Check sheet for the modelled part. Datum: model origin and axes. Units: mm. A direction names the side the tool comes from. Coordinates: 2 decimals unless noted, no trailing zeros. Loops run counter-clockwise (first coordinate to the right, second up) from the corner with the lowest first, then second, coordinate; pieces in that order, holes last. Notation, with made-up numbers: M -25.5,77.25 L 22.5,77.25 A11 ccw 22.5,96.25 Z; hole C 8.25,3.5 d10. An arc over 180 degrees is marked long. Return JSON: item names as keys, results as strings.
from build123d import *

# Parameters (mm, degrees)
PAD003_DEPTH    = 30
SKETCH011_R     = 4.25
PAD004_DEPTH    = 2
SKETCH012_R     = 4.25
PAD005_DEPTH    = 2
SKETCH008_R     = 2.5
POCKET001_DEPTH = 28.501
SKETCH009_R     = 4.75
POCKET002_DEPTH = 28.501
SKETCH010_R     = 2.5
POCKET003_DEPTH = 48.111


with BuildPart() as part:
    # Sketch007 → Pad003 (new body, symmetric)
    with BuildSketch(Plane(origin=(0, 0, 10), x_dir=(0, 1, 0), z_dir=(1, 0, 0))):
        with BuildLine():
            Line((-12, 6.09), (-28.5, 6.09))
            Line((-28.5, 6.09), (-28.5, 14.09))
            Line((-28.5, 14.09), (-19.722169, 14.09))
            ThreePointArc((-14.09, 19.722169), (-17.656854, 17.656854), (-19.722169, 14.09))
            Line((-14.09, 19.722169), (-14.09, 34.02))
            ThreePointArc((0, 48.11), (-9.963135, 43.983135), (-14.09, 34.02))
            Line((0, 48.11), (0, 34.02))
            Line((0, 34.02), (-6.09, 34.02))
            Line((-6.09, 34.02), (-6.09, 12))
            Line((-12, 12), (-6.09, 12))
            Line((-12, 6.09), (-12, 12))
        make_face()
    pad003 = extrude(amount=PAD003_DEPTH, both=True)

    # Mirrored: Pad003 across Sketch007 V_Axis
    add(pad003.mirror(Plane(origin=(0, 0, 10), x_dir=(1, 0, 0), z_dir=(0, 1, 0))))

    # Sketch011 → Pad004 (join)
    with BuildSketch(Plane.XY.offset(15.085)):
        with Locations((-15, 20.35)):
            Circle(SKETCH011_R)
        with Locations((15, 20.35)):
            Circle(SKETCH011_R)
        with Locations((15, -20.35)):
            Circle(SKETCH011_R)
        with Locations((-15, -20.35)):
            Circle(SKETCH011_R)
    extrude(amount=PAD004_DEPTH)

    # Sketch012 → Pad005 (join)
    with BuildSketch(Plane(origin=(0, 5.085, 30.35), x_dir=(1, 0, 0), z_dir=(0, -1, 0))):
        with Locations((-15, 0)):
            Circle(SKETCH012_R)
        with Locations((15, 0)):
            Circle(SKETCH012_R)
    extrude(amount=-PAD005_DEPTH)

    # Sketch008 → Pocket001 (cut, through all)
    with BuildSketch(Plane(origin=(0, 0, 30.35), x_dir=(1, 0, 0), z_dir=(0, -1, 0))):
        with Locations((-15, 0)):
            Circle(SKETCH008_R)
        with Locations((15, 0)):
            Circle(SKETCH008_R)
    extrude(amount=-POCKET001_DEPTH, mode=Mode.SUBTRACT)

    # Sketch009 → Pocket002 (cut, through all)
    with BuildSketch(Plane(origin=(0, 0, 30.35), x_dir=(1, 0, 0), z_dir=(0, -1, 0))):
        with Locations((-15, 0)):
            Circle(SKETCH009_R)
        with Locations((15, 0)):
            Circle(SKETCH009_R)
    extrude(amount=POCKET002_DEPTH, mode=Mode.SUBTRACT)

    # Sketch010 → Pocket003 (cut, through all)
    with BuildSketch(Plane.XY.offset(10)):
        with Locations((-15, 20.35)):
            Circle(SKETCH010_R)
        with Locations((15, 20.35)):
            Circle(SKETCH010_R)
        with Locations((15, -20.35)):
            Circle(SKETCH010_R)
        with Locations((-15, -20.35)):
            Circle(SKETCH010_R)
    extrude(amount=POCKET003_DEPTH, mode=Mode.SUBTRACT)


solid = part.part
1) Set-up check for faces 1 (the face through (14.447, -16.136, 15.58)), 2 (the face through (0, 24, 24.09)), 3 (the face through (18, 5.085, 30)): record each of +Z, -Z, +X, -X, +Y, -Y from which the full face is reachable in a straight line by a thin tool's end or side.
Answers:
{"face 1": "-Z", "face 2": "+Z, +X, -X, +Y", "face 3": "-Z, +X, -X, -Y"}
2) Section check C-C on z = 32. Count the separate pieces of the cut face and the enclosed holes in it, then the cut area to 3 significant figures.
Answers:
{"separate pieces": "6", "enclosed holes": "0", "area": "766 mm²"}
3) Scan lines: line 1 along X through (y, z) = (20.35, 21.5); line 2 along Y through (x, z) = (-15, 22.5); line 3 along Y through (x, z) = (-15, 17.5). Record each from-to range of solid material in increasing order. Write a range as [from, to].
Answers:
{"line 1": "[-30, -17.5], [-12.5, 12.5], [17.5, 30]", "line 2": "[-28.5, -22.85], [-17.85, -6.09], [6.09, 17.85], [22.85, 28.5]", "line 3": "[-28.5, -22.85], [-17.85, -12], [12, 17.85], [22.85, 28.5]"}
4) Go/stop test with flat-tipped pins: pin 1 Ø12 at (y, z) = (22.5, 41) entering from -X; pin 2 Ø1.5 at (x, y) = (17.5, 14.5) entering from -Z; pin 3 Ø15.5 at (x, z) = (5, 37) entering from +Y; pin 4 Ø8.5 at (x, z) = (-15, 30.35) entering from +Y. Record where each tip stops, or that it passes through.
Answers:
{"pin 1": "through", "pin 2": "z = 16.09", "pin 3": "y = 15.38", "pin 4": "y = 18.61"}
5) Section check A-A on z = 18. Record the cut outline in (x, y), then the cut area to 3 significant figures.
Answers:
{"outline": "M -30,-28.5 L 30,-28.5 L 30,-12 L -30,-12 Z; M -30,12 L 30,12 L 30,28.5 L -30,28.5 Z; hole C -15,-20.35 d5; hole C -15,20.35 d5; hole C 15,-20.35 d5; hole C 15,20.35 d5", "area": "1,900 mm²"}
6) Section check B-B on x = 3. Record the cut outline in (y, z), then the cut area to 3 significant figures.
Answers:
{"outline": "M -28.5,16.09 L -12,16.09 L -12,22 L -6.09,22 L -6.09,44.02 L 6.09,44.02 L 6.09,22 L 12,22 L 12,16.09 L 28.5,16.09 L 28.5,24.09 L 19.72,24.09 A8 ccw 14.09,29.72 L 14.09,44.02 A14.09 ccw 0,58.11 A14.09 ccw -14.09,44.02 L -14.09,29.72 A8 ccw -19.72,24.09 L -28.5,24.09 Z", "area": "963 mm²"}
7) Draft check along X on faces 4 (the face through (0, 14.09, 37)), 5 (the face through (14.447, 24.564, 15.58)), 6 (the face through (-30, -7, 33)). Enter one of: +X half, -X half, draft (parallel to the pull), parting line (faces both ways), or undercut.
Answers:
{"face 4": "draft", "face 5": "undercut", "face 6": "-X half"}
